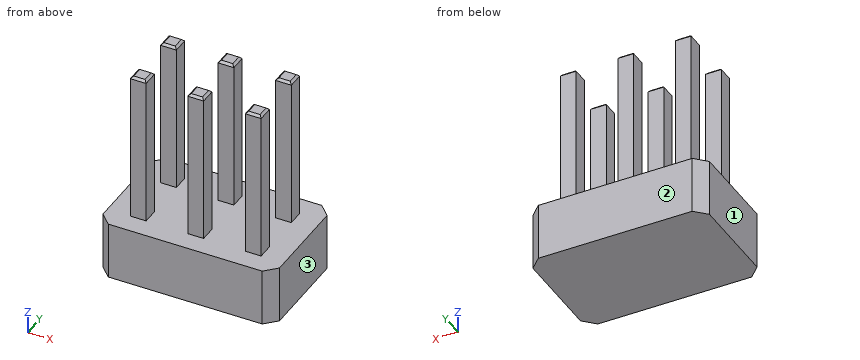
```python
from build123d import *

# Parameters (mm, degrees)
SKETCH1_W           = 7.8
SKETCH1_H           = 5
BOSS_EXTRUDE1_DEPTH = 2.54
SKETCH2_W           = 0.7
SKETCH2_H           = 0.7
BOSS_EXTRUDE2_DEPTH = 6.7
CHAMFER1_SIZE       = 0.5
CHAMFER2_SIZE       = 0.1


with BuildPart() as part:
    # Sketch1 → Boss-Extrude1 (new body)
    with BuildSketch(Plane.XY):
        Rectangle(SKETCH1_W, SKETCH1_H)
    extrude(amount=BOSS_EXTRUDE1_DEPTH)

    # Sketch2 → Boss-Extrude2 (add)
    with BuildSketch(Plane.XY.offset(2.54)):
        with Locations((0, 1.27)):
            Rectangle(SKETCH2_W, SKETCH2_H)
        with Locations((-2.54, 1.27)):
            Rectangle(SKETCH2_W, SKETCH2_H)
        with Locations((2.54, 1.27)):
            Rectangle(SKETCH2_W, SKETCH2_H)
        with Locations((0, -1.27)):
            Rectangle(SKETCH2_W, SKETCH2_H)
        with Locations((2.54, -1.27)):
            Rectangle(SKETCH2_W, SKETCH2_H)
        with Locations((-2.54, -1.27)):
            Rectangle(SKETCH2_W, SKETCH2_H)
    extrude(amount=BOSS_EXTRUDE2_DEPTH)

    # Chamfer1
    chamfer1_edges = [part.edges().sort_by_distance(p)[0] for p in [
        (3.9, -2.5, 1.27),
        (-3.9, -2.5, 1.27),
        (-3.9, 2.5, 1.27),
        (3.9, 2.5, 1.27),
    ]]
    chamfer(chamfer1_edges, length=CHAMFER1_SIZE)

    # Chamfer2
    chamfer2_edges = [part.edges().sort_by_distance(p)[0] for p in [
        (-2.89, 1.27, 9.24),
        (-2.54, 0.92, 9.24),
        (-2.19, 1.27, 9.24),
        (-2.54, 1.62, 9.24),
        (-0.35, 1.27, 9.24),
        (0, 0.92, 9.24),
        (0.35, 1.27, 9.24),
        (0, 1.62, 9.24),
        (2.19, 1.27, 9.24),
        (2.54, 0.92, 9.24),
        (2.89, 1.27, 9.24),
        (2.54, 1.62, 9.24),
        (-0.35, -1.27, 9.24),
        (0, -1.62, 9.24),
        (0.35, -1.27, 9.24),
        (0, -0.92, 9.24),
        (2.19, -1.27, 9.24),
        (2.54, -1.62, 9.24),
        (2.89, -1.27, 9.24),
        (2.54, -0.92, 9.24),
        (-2.89, -1.27, 9.24),
        (-2.54, -1.62, 9.24),
        (-2.19, -1.27, 9.24),
        (-2.54, -0.92, 9.24),
    ]]
    chamfer(chamfer2_edges, length=CHAMFER2_SIZE)


solid = part.part
```
Can you work these out from the model? Positions are in its coordinate system, mm. Face numbers are marked on the shaded views. Coordinates: 2 decimals unless noted, no trailing zeros. Order: outer loops, then holes, each group sorted by start corner. A loop starts at its lowest first (then second) coordinate and runs counter-clockwise, first axis right, second up.
1. I need wall thicknesses on line 1 (X direction, y = -1.5, z = 7.25); line 2 (Y direction, x = -2.5, z = 8.25); line 3 (Z direction, x = -0.5, y = 1.7). Which ranges of each line are inside material? Lowest first, please.
2. If we section it at D-D (x = -2): Please give me the cut outline in (y, z).
3. Thinking about a two-plate mould opening in X: for the marked faces 1, 2 and 3, which applies, +X half, -X half, draft (parallel to the pull), parting line (faces both ways), or undercut?
4. If we section it at A-A (z = 6): Please give me the cut outline in (x, y), then the cut area to 3 significant figures.
5. I'm going to push flat-ended pins straight in: pin 1 (3 mm diameter, centred on x = -2, z = 8, fed in from -Y); pin 2 (0.6 mm diameter, centred on x = -2.5, z = 4.5, fed in from +Y); pin 3 (0.8 mm diameter, centred on y = 1.5, z = 5, fed in from +X). Where does each tip first touch, or does it pass through?
6. If we section it at C-C (x = 0): Please give me the cut outline in (y, z).
7. If we section it at B-B (y = 1.15): Please give me the cut outline in (x, z), then the cut area to 3 significant figures.
Entries:
1. line 1: x = -2.89 to -2.19, -0.35 to 0.35, 2.19 to 2.89
1. line 2: y = -1.62 to -0.92, 0.92 to 1.62
1. line 3: z = 0 to 2.54
2. outline: (-2.5, 0) - (2.5, 0) - (2.5, 2.54) - (-2.5, 2.54) - close
3. face 1: -X half
3. face 2: draft
3. face 3: +X half
4. outline: (-2.89, -1.62) - (-2.19, -1.62) - (-2.19, -0.92) - (-2.89, -0.92) - close; (-2.89, 0.92) - (-2.19, 0.92) - (-2.19, 1.62) - (-2.89, 1.62) - close; (-0.35, -1.62) - (0.35, -1.62) - (0.35, -0.92) - (-0.35, -0.92) - close; (-0.35, 0.92) - (0.35, 0.92) - (0.35, 1.62) - (-0.35, 1.62) - close; (2.19, -1.62) - (2.89, -1.62) - (2.89, -0.92) - (2.19, -0.92) - close; (2.19, 0.92) - (2.89, 0.92) - (2.89, 1.62) - (2.19, 1.62) - close
4. area: 2.94 mm2
5. pin 1: stops at y = -1.62
5. pin 2: stops at y = 1.62
5. pin 3: stops at x = 2.89
6. outline: (-2.5, 0) - (2.5, 0) - (2.5, 2.54) - (1.62, 2.54) - (1.62, 9.14) - (1.52, 9.24) - (1.02, 9.24) - (0.92, 9.14) - (0.92, 2.54) - (-0.92, 2.54) - (-0.92, 9.14) - (-1.02, 9.24) - (-1.52, 9.24) - (-1.62, 9.14) - (-1.62, 2.54) - (-2.5, 2.54) - close
7. outline: (-3.9, 0) - (3.9, 0) - (3.9, 2.54) - (2.89, 2.54) - (2.89, 9.14) - (2.79, 9.24) - (2.29, 9.24) - (2.19, 9.14) - (2.19, 2.54) - (0.35, 2.54) - (0.35, 9.14) - (0.25, 9.24) - (-0.25, 9.24) - (-0.35, 9.14) - (-0.35, 2.54) - (-2.19, 2.54) - (-2.19, 9.14) - (-2.29, 9.24) - (-2.79, 9.24) - (-2.89, 9.14) - (-2.89, 2.54) - (-3.9, 2.54) - close
7. area: 33.9 mm2
